Input: part model. Units: mm. Frame: model coordinates. A direction names the side the tool comes from. Round coordinates to 2 decimals unless told otherwise and drop trailing zeros. Write each loop counter-clockwise with the first axis right and the second up, starting at its lowest first coordinate (ties: lowest second). Pieces come first, ordered by that corner, then holes. Notation, with made-up numbers: (28.5, 14) -> (32.5, 14) arc R12 ccw to (32.5, 37) -> close; hole circle Ø6 at (27.25, 79). An arc over 180 degrees is marked (long way). Write item = value, one per line. Start each with the question number.
```python
from build123d import *

# Parameters (mm, degrees)
SKETCH_1_W                      = 400
SKETCH_1_H                      = 400
EXTRUDE_1_DEPTH                 = 42
CHAMFER_1_SIZE                  = 30
CUT_EXTRUDE_1_DEPTH             = 450.181477802
PATTERN_CIRCULAR_1_COUNT        = 2
PATTERN_CIRCULAR_1_ANGLE        = 90
PATTERN_CIRCULAR_1_COPY_1_DEPTH = 450.181477802
HOLE_WIZARD_1_D                 = 13
HOLE_WIZARD_1_CBORE_D           = 23
HOLE_WIZARD_1_CBORE_DEPTH       = 14


with BuildPart() as part:
    # Sketch 1 → Extrude 1 (new body)
    with BuildSketch(Plane.XY):
        Rectangle(SKETCH_1_W, SKETCH_1_H)
    extrude(amount=EXTRUDE_1_DEPTH)

    # Chamfer 1
    chamfer_1_edges = [part.edges().sort_by_distance(p)[0] for p in [
        (200, -200, 21),
        (-200, -200, 21),
        (-200, 200, 21),
        (200, 200, 21),
    ]]
    chamfer(chamfer_1_edges, length=CHAMFER_1_SIZE)

    # Sketch 2 → Cut-Extrude 1 (cut, symmetric)
    with BuildSketch(Plane.XZ.offset(200)):
        Polygon((-142, 21), (-106, 21), (-113, 42), (-135, 42), align=None)
    cut_extrude_1 = extrude(amount=CUT_EXTRUDE_1_DEPTH, both=True, mode=Mode.SUBTRACT)

    # Mirror 1: Cut-Extrude 1 across plane
    add(cut_extrude_1.mirror(Plane(origin=(0, 0, 0), x_dir=(0, 0, 1), z_dir=(1, 0, 0))), mode=Mode.SUBTRACT)

    # Pattern Circular 1: Cut-Extrude 1 ×2 about axis
    pattern_circular_1_axis = Axis((0, 0, -2.1), (0, 0, 1))
    for i in range(1, PATTERN_CIRCULAR_1_COUNT):
        add(cut_extrude_1.rotate(pattern_circular_1_axis, i * PATTERN_CIRCULAR_1_ANGLE / (PATTERN_CIRCULAR_1_COUNT - 1)), mode=Mode.SUBTRACT)

    # Pattern Circular 1 copy 1 sketch → Pattern Circular 1 copy 1 (cut, symmetric)
    with BuildSketch(Plane(origin=(200, 0, 0), x_dir=(0, -1, 0), z_dir=(1, 0, 0))):
        Polygon((-142, -21), (-106, -21), (-113, -42), (-135, -42), align=None)
    extrude(amount=PATTERN_CIRCULAR_1_COPY_1_DEPTH, both=True, mode=Mode.SUBTRACT)

    # Hole Wizard 1 (through all)
    with Locations(Plane.XY.offset(42)):
        with Locations((0, 0), (95, 89), (95, -89), (-95, -89), (-95, 89)):
            CounterBoreHole(HOLE_WIZARD_1_D / 2, HOLE_WIZARD_1_CBORE_D / 2, HOLE_WIZARD_1_CBORE_DEPTH)


solid = part.part
```
1. Section B-B (y = -89). Output: boundary loops of the cut face in (x, z), then the cut area to 3 significant figures.
2. Reachability of faces 1 (the flat face through (1.58, -109.45, 31.35)), 2 (the flat face through (109.45, 167.04, 31.35)), 3 (the cylindrical face through (-97.493, 77.773, 35.098)), 4 (the flat face through (-131, 3, 21)) from +Z, -Z, +X, -X, +Y, -Y: full face, straight path, thin tool, end or side. Return the list, or none.
3. Pin query (flat end, axial travel): P1, Ø20.5, axis at x = 95, y = -89, coming from the -Z side; P2, Ø20.5, axis at x = -95, y = -89, coming from the +Z side. Return the tip coordinate at first contact, or that it passes through.
4. Section D-D (x = -95). Output: boundary loops of the cut face in (y, z).
5. Section A-A (x = 0). Output: boundary loops of the cut face in (y, z), then the cut area to 3 significant figures.
6. Line query: line 1 along Y through (x, z) = (-95, 18); line 2 along Y through (x, z) = (0, 7.5); line 3 along Y through (x, z) = (155.5, 26). Output: solid intervals per line, ascending.
7. Section C-C (z = 9). Output: boundary loops of the cut face in (x, y), then the cut area to 3 significant figures.
8. Mould query, pull axis X, two halves, no side actions, for faces 5 (the flat face through (-185, -185, 21)), 6 (the flat face through (-138.45, 167.04, 31.65)), 7 (the flat face through (42, 3, 0)). Classes: pulls with the +X half, pulls with the -X half, needs draft (parallel to the pull), parting line crosses it, or undercut.
Check sheet entries:
q1.outline = (-200, 0) -> (-101.5, 0) -> (-101.5, 28) -> (-106.5, 28) -> (-106.5, 42) -> (-113, 42) -> (-106, 21) -> (-142, 21) -> (-135, 42) -> (-200, 42) -> close; (-88.5, 0) -> (88.5, 0) -> (88.5, 28) -> (83.5, 28) -> (83.5, 42) -> (-83.5, 42) -> (-83.5, 28) -> (-88.5, 28) -> close; (101.5, 0) -> (200, 0) -> (200, 42) -> (135, 42) -> (142, 21) -> (106, 21) -> (113, 42) -> (106.5, 42) -> (106.5, 28) -> (101.5, 28) -> close
q1.area = 14,200 mm2
q2.face_1 = +X, -X
q2.face_2 = +Y, -Y
q2.face_3 = +Z
q2.face_4 = none
q3.P1 = 0
q3.P2 = 28
q4.outline = (-200, 0) -> (-95.5, 0) -> (-95.5, 28) -> (-100.5, 28) -> (-100.5, 42) -> (-113, 42) -> (-106, 21) -> (-142, 21) -> (-135, 42) -> (-200, 42) -> close; (-82.5, 0) -> (82.5, 0) -> (82.5, 28) -> (77.5, 28) -> (77.5, 42) -> (-77.5, 42) -> (-77.5, 28) -> (-82.5, 28) -> close; (95.5, 0) -> (200, 0) -> (200, 42) -> (135, 42) -> (142, 21) -> (106, 21) -> (113, 42) -> (100.5, 42) -> (100.5, 28) -> (95.5, 28) -> close
q5.outline = (-200, 0) -> (-6.5, 0) -> (-6.5, 28) -> (-11.5, 28) -> (-11.5, 42) -> (-113, 42) -> (-106, 21) -> (-142, 21) -> (-135, 42) -> (-200, 42) -> close; (6.5, 0) -> (200, 0) -> (200, 42) -> (135, 42) -> (142, 21) -> (106, 21) -> (113, 42) -> (11.5, 42) -> (11.5, 28) -> (6.5, 28) -> close
q5.area = 14,900 mm2
q6.line_1 = -200 to -95.5, -82.5 to 82.5, 95.5 to 200
q6.line_2 = -200 to -6.5, 6.5 to 200
q6.line_3 = -200 to -140.33, -107.67 to 107.67, 140.33 to 200
q7.outline = (-200, -170) -> (-170, -200) -> (170, -200) -> (200, -170) -> (200, 170) -> (170, 200) -> (-170, 200) -> (-200, 170) -> close; hole circle Ø13 at (-95, -89); hole circle Ø13 at (-95, 89); hole circle Ø13 at (0, 0); hole circle Ø13 at (95, -89); hole circle Ø13 at (95, 89)
q7.area = 158,000 mm2
q8.face_5 = pulls with the -X half
q8.face_6 = undercut
q8.face_7 = needs draft
